```python
from build123d import *

# Parameters (mm, degrees)
F0_W     = 54.104183
F0_H     = 44.93398
F1_DEPTH = 161.07251
F4_D     = 25.4
F5_D     = 25.4


with BuildPart() as f1:
    # F0 (on Front) → F1 (new body)
    with BuildSketch(Plane.XZ):
        with Locations((-42.297548, 38.514842)):
            Rectangle(F0_W, F0_H)
    extrude(amount=F1_DEPTH)

    # F4 (through all)
    with Locations(Plane.XZ.offset(161.07251)):
        with Locations((-47.465287, 36.99689)):
            Hole(F4_D / 2)

    # F5 (through all)
    with Locations(Plane.XZ.offset(161.07251)):
        with Locations((-31.359639, 45.062546)):
            Hole(F5_D / 2)


solid = f1.part
```
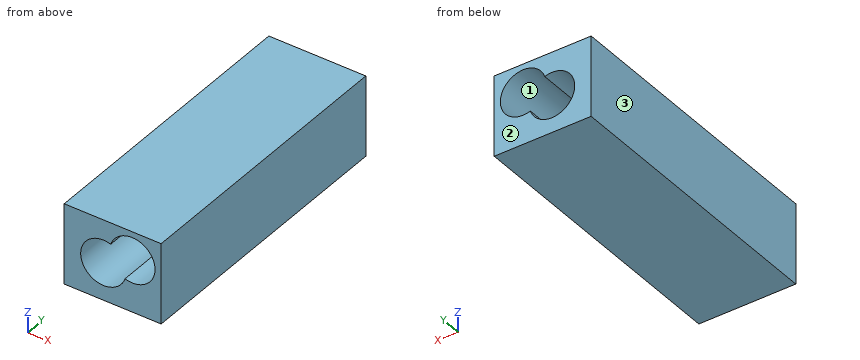
CAD build for the part. Positions are in the model's coordinates, mm. Face numbers are marked on the shaded views. Coordinates: 2 decimals unless noted, no trailing zeros. Write each loop counter-clockwise with the first axis right and the second up, starting at its lowest first coordinate (ties: lowest second). Pieces come first, ordered by that corner, then holes.
(1) Cut at C-C, the plane y = -15.5. List the corners of the cut face in (x, z).
(2) Two-plate mould, pull along X, no slides. Class the marked faces 1, 2 and 3: +X half, -X half, draft (parallel to the pull), parting line (faces both ways), or undercut.
(3) Cut at A-A, the plane z = 43.5. List the corners of the cut face in (x, y), and give its area (3 significant figures).
(4) Drill centre lines: probe 1 along X at (y, z) = (-143, 56.5); probe 2 along X at (y, z) = (-121, 28); probe 3 along Z at (x, y) = (-42, -109). Where is each one in solid material? Low to high.
(5) Cut at B-B, the plane x = -31.5. List the corners of the cut face in (y, z), and give its area (3 significant figures).
Geometry says:
1. outline: (-69.35, 16.05) - (-15.25, 16.05) - (-15.25, 60.98) - (-69.35, 60.98) - close; hole (-43.42, 49.04) arc R12.7 ccw (long way) to (-35.4, 33.02) arc R12.7 ccw (long way) to start
2. face 1: undercut
2. face 2: draft
2. face 3: -X half
3. outline: (-69.35, -161.07) - (-58.37, -161.07) - (-58.37, 0) - (-69.35, 0) - close; (-18.76, -161.07) - (-15.25, -161.07) - (-15.25, 0) - (-18.76, 0) - close
3. area: 2,330 mm2
4. probe 1: x = -69.35 to -36.88, -25.84 to -15.25
4. probe 2: x = -69.35 to -56.43, -38.5 to -15.25
4. probe 3: z = 16.05 to 25.53, 52 to 60.98
5. outline: (-161.07, 16.05) - (0, 16.05) - (0, 32.36) - (-161.07, 32.36) - close; (-161.07, 57.76) - (0, 57.76) - (0, 60.98) - (-161.07, 60.98) - close
5. area: 3,150 mm2
